Here's how the part is built. I have some questions about the finished solid (model axes, mm). A direction names the side the tool comes from. Coordinates: 2 decimals unless noted, no trailing zeros. Write each loop counter-clockwise with the first axis right and the second up, starting at its lowest first coordinate (ties: lowest second). Pieces come first, ordered by that corner, then holes. Notation, with made-up numbers: M -23,-34 L 8,-34 A27 ccw 8,-4 Z; hole C 11.25,27.25 d5. An arc over 180 degrees is marked long. Use one line per item in the form item = value. Start each with the question number.
1. I want a section at A-A, the plane z = -0.5. List the corners of the cut face in (x, y) for me, plus the area to 3 significant figures.
2. Thinking about a two-plate mould opening in Z: for faces 1 (the face through (-6, 3, -9.5)), 2 (the face through (-6, -3, 1.1)), 3 (the face through (-7.134, -3.724, -8.493)), 4 (the face through (5.95, 4.087, 0.846)), which applies, released by +Z, released by -Z, zero draft, split by the parting line, or undercut?
3. I want a section at B-B, the plane y = 0. List the corners of the cut face in (x, z) for me.
4. On a 3-axis mill with a long thin cutter (end or side, diameter ignored), from which of +Z, -Z, +X, -X, +Y, -Y can I reach the whole of each face in a straight line? I mean faces 5 (the face through (0, -8.2, -6)), 6 (the face through (-5.95, -4.087, 0.846)), 7 (the face through (7.134, -3.724, -0.211)). Say none if no direction works.
5. I want a section at C-C, the plane x = 0. List the corners of the cut face in (y, z) for me, plus the area to 3 significant figures.
6. I'm going to push flat-ended pins straight in: pin 1 Ø1 at (x, z) = (6, -5.5) entering from +Y; pin 2 Ø1.5 at (x, z) = (-3, -5.5) entering from -Y; pin 3 Ø1 at (y, z) = (3, -4) entering from +X. Where does each tip first touch, or does it pass through?
7. I want a section at D-D, the plane z = -4.5. List the corners of the cut face in (x, y) for me.
8. Please list where these lines run through material, in increasing order: line 1 along X through (y, z) = (-0.75, -7.75); line 2 along X through (y, z) = (-2.75, -2.5); line 3 along Y through (x, z) = (4.75, -4). Write a range as [from, to].
from build123d import *

# Parameters (mm, degrees)
SKETCH007_R                    = 8.5
PAD006_DEPTH                   = 7
THICKNESS_T                    = -0.5
PAD007_DEPTH                   = 1.6
PAD007_POLARPATTERN_2_DEPTH    = 1.6
PAD008_DEPTH                   = 0.5
PAD008_POLARPATTERN001_2_DEPTH = 0.5
SKETCH011_W                    = 13.925584
SKETCH011_H                    = 6.6246
POCKET001_DEPTH                = 2
SKETCH013_W                    = 13.925584
SKETCH013_H                    = 6.6246
POCKET002_DEPTH                = 2
SKETCH014_R                    = 8
POCKET003_DEPTH                = 0.5
PAD009_DEPTH                   = 1
PAD009_MIRRORED002_2_DEPTH     = 1
PAD010_DEPTH                   = 0.5
PAD010_MIRRORED004_2_DEPTH     = 0.5
FILLET_R                       = 0.5


with BuildPart() as part:
    # Sketch007 (on DatumPlane) → Pad006 (new body)
    with BuildSketch(Plane(origin=(0, 0, -1), x_dir=(1, 0, 0), z_dir=(0, 0, -1))):
        Circle(SKETCH007_R)
    extrude(amount=PAD006_DEPTH)

    # Thickness
    thickness_openings = [part.faces().sort_by_distance(p)[0] for p in [
        (0, 0, -1),
    ]]
    offset(amount=THICKNESS_T, openings=thickness_openings)

    # Sketch008 (on Face3 of Thickness) → Pad007 (join)
    with BuildSketch(Plane.XY.offset(-1)):
        with BuildLine():
            ThreePointArc((-7.005526, 4.813794), (-7.541696, 3.920819), (-7.964623, 2.96897))
            Line((-7.540357, 2.810816), (-7.964623, 2.96897))
            ThreePointArc((-6.632349, 4.557368), (-7.139959, 3.711961), (-7.540357, 2.810816))
            Line((-6.632349, 4.557368), (-7.005526, 4.813794))
        make_face()
    pad007 = extrude(amount=PAD007_DEPTH)

    # Sketch008 PolarPattern 2 → Pad007 PolarPattern 2 (add)
    with BuildSketch(Plane(origin=(0, 0, -1), x_dir=(-1, 0, 0), z_dir=(0, 0, 1))):
        with BuildLine():
            ThreePointArc((-7.005526, 4.813794), (-7.541696, 3.920819), (-7.964623, 2.96897))
            Line((-7.540357, 2.810816), (-7.964623, 2.96897))
            ThreePointArc((-6.632349, 4.557368), (-7.139959, 3.711961), (-7.540357, 2.810816))
            Line((-6.632349, 4.557368), (-7.005526, 4.813794))
        make_face()
    pad007_polarpattern_2 = extrude(amount=PAD007_POLARPATTERN_2_DEPTH)

    # Mirrored: Pad007, Pad007 PolarPattern 2 across Sketch008 V_Axis
    add(pad007.mirror(Plane(origin=(0, 0, -1), x_dir=(0, 0, 1), z_dir=(1, 0, 0))))
    add(pad007_polarpattern_2.mirror(Plane(origin=(0, 0, -1), x_dir=(0, 0, 1), z_dir=(1, 0, 0))))

    # Sketch009 (on Face23 of MultiTransform) → Pad008 (join)
    with BuildSketch(Plane.XY.offset(0.6)):
        with BuildLine():
            ThreePointArc((-7.005526, 4.813794), (-7.542066, 3.921011), (-7.964623, 2.96897))
            Line((-5.09111, 1.862853), (-7.964623, 2.96897))
            ThreePointArc((-4.469489, 3.068188), (-4.818529, 2.485236), (-5.09111, 1.862853))
            Line((-7.005526, 4.813794), (-4.469489, 3.068188))
        make_face()
    pad008 = extrude(amount=PAD008_DEPTH)

    # Sketch009 PolarPattern001 2 → Pad008 PolarPattern001 2 (add)
    with BuildSketch(Plane(origin=(0, 0, 0.6), x_dir=(-1, 0, 0), z_dir=(0, 0, 1))):
        with BuildLine():
            ThreePointArc((-7.005526, 4.813794), (-7.542066, 3.921011), (-7.964623, 2.96897))
            Line((-5.09111, 1.862853), (-7.964623, 2.96897))
            ThreePointArc((-4.469489, 3.068188), (-4.818529, 2.485236), (-5.09111, 1.862853))
            Line((-7.005526, 4.813794), (-4.469489, 3.068188))
        make_face()
    pad008_polarpattern001_2 = extrude(amount=PAD008_POLARPATTERN001_2_DEPTH)

    # Mirrored001: Pad008, Pad008 PolarPattern001 2 across Sketch009 V_Axis
    add(pad008.mirror(Plane(origin=(0, 0, 0.6), x_dir=(0, 0, 1), z_dir=(1, 0, 0))))
    add(pad008_polarpattern001_2.mirror(Plane(origin=(0, 0, 0.6), x_dir=(0, 0, 1), z_dir=(1, 0, 0))))

    # Sketch011 (on Face1 of ShapeBinder001) → Pocket001 (cut)
    with BuildSketch(Plane(origin=(0, 0, -1), x_dir=(1, 0, 0), z_dir=(0, 0, -1))):
        with Locations((0, 8.1877)):
            Rectangle(SKETCH011_W, SKETCH011_H)
    extrude(amount=POCKET001_DEPTH, mode=Mode.SUBTRACT)

    # Sketch013 → Pocket002 (cut)
    with BuildSketch(Plane.XY.offset(-8)):
        with Locations((0, -8.1877)):
            Rectangle(SKETCH013_W, SKETCH013_H)
    extrude(amount=POCKET002_DEPTH, mode=Mode.SUBTRACT)

    # Sketch014 → Pocket003 (cut)
    with BuildSketch(Plane.XY.offset(-8)):
        Circle(SKETCH014_R)
    extrude(amount=POCKET003_DEPTH, mode=Mode.SUBTRACT)

    # Sketch012 → Pad009 (join)
    with BuildSketch(Plane.XY.offset(-8)):
        with BuildLine():
            ThreePointArc((-7.005526, 4.813794), (-7.541696, 3.920819), (-7.964623, 2.96897))
            Line((-7.540357, 2.810816), (-7.964623, 2.96897))
            ThreePointArc((-6.632349, 4.557368), (-7.139959, 3.711961), (-7.540357, 2.810816))
            Line((-6.632349, 4.557368), (-7.005526, 4.813794))
        make_face()
    pad009 = extrude(amount=-PAD009_DEPTH)

    # Sketch012 Mirrored002 2 → Pad009 Mirrored002 2 (add)
    with BuildSketch(Plane(origin=(0, 0, -8), x_dir=(-1, 0, 0), z_dir=(0, 0, -1))):
        with BuildLine():
            ThreePointArc((-7.005526, 4.813794), (-7.541696, 3.920819), (-7.964623, 2.96897))
            Line((-7.540357, 2.810816), (-7.964623, 2.96897))
            ThreePointArc((-6.632349, 4.557368), (-7.139959, 3.711961), (-7.540357, 2.810816))
            Line((-6.632349, 4.557368), (-7.005526, 4.813794))
        make_face()
    pad009_mirrored002_2 = extrude(amount=PAD009_MIRRORED002_2_DEPTH)

    # Mirrored003: Pad009, Pad009 Mirrored002 2 across Sketch012 H_Axis
    add(pad009.mirror(Plane(origin=(0, 0, -8), x_dir=(0, 0, 1), z_dir=(0, 1, 0))))
    add(pad009_mirrored002_2.mirror(Plane(origin=(0, 0, -8), x_dir=(0, 0, 1), z_dir=(0, 1, 0))))

    # Sketch015 → Pad010 (join)
    with BuildSketch(Plane.XY.offset(-9.5)):
        with BuildLine():
            ThreePointArc((-7.005526, 4.813794), (-7.542066, 3.921011), (-7.964623, 2.96897))
            Line((-5.09111, 1.862853), (-7.964623, 2.96897))
            ThreePointArc((-4.469489, 3.068188), (-4.818529, 2.485236), (-5.09111, 1.862853))
            Line((-7.005526, 4.813794), (-4.469489, 3.068188))
        make_face()
    pad010 = extrude(amount=PAD010_DEPTH)

    # Sketch015 Mirrored004 2 → Pad010 Mirrored004 2 (add)
    with BuildSketch(Plane(origin=(0, 0, -9.5), x_dir=(-1, 0, 0), z_dir=(0, 0, -1))):
        with BuildLine():
            ThreePointArc((-7.005526, 4.813794), (-7.542066, 3.921011), (-7.964623, 2.96897))
            Line((-5.09111, 1.862853), (-7.964623, 2.96897))
            ThreePointArc((-4.469489, 3.068188), (-4.818529, 2.485236), (-5.09111, 1.862853))
            Line((-7.005526, 4.813794), (-4.469489, 3.068188))
        make_face()
    pad010_mirrored004_2 = extrude(amount=-PAD010_MIRRORED004_2_DEPTH)

    # Mirrored005: Pad010, Pad010 Mirrored004 2 across Sketch015 H_Axis
    add(pad010.mirror(Plane(origin=(0, 0, -9.5), x_dir=(0, 0, 1), z_dir=(0, 1, 0))))
    add(pad010_mirrored004_2.mirror(Plane(origin=(0, 0, -9.5), x_dir=(0, 0, 1), z_dir=(0, 1, 0))))

    # Fillet
    fillet_edges = [part.edges().sort_by_distance(p)[0] for p in [
        (-4.469489, 3.068188, 0.85),
        (-5.09111, 1.862853, 0.85),
        (-5.09111, -1.862853, 0.85),
        (-4.469489, -3.068188, 0.85),
        (4.469489, 3.068188, 0.85),
        (5.09111, 1.862853, 0.85),
        (5.09111, -1.862853, 0.85),
        (4.469489, -3.068188, 0.85),
        (-4.469489, 3.068188, -9.25),
        (-5.09111, 1.862853, -9.25),
        (4.469489, 3.068188, -9.25),
        (5.09111, 1.862853, -9.25),
        (-5.09111, -1.862853, -9.25),
        (-4.469489, -3.068188, -9.25),
        (5.09111, -1.862853, -9.25),
        (4.469489, -3.068188, -9.25),
    ]]
    fillet(fillet_edges, radius=FILLET_R)


solid = part.part
Answer list:
q1.outline = M -7.96,-2.97 A8.5 ccw -7.01,-4.81 L -6.63,-4.56 A8.05 cw -7.54,-2.81 Z; M -7.96,2.97 L -7.54,2.81 A8.05 cw -6.63,4.56 L -7.01,4.81 A8.5 ccw Z; M 6.63,-4.56 L 7.01,-4.81 A8.5 ccw 7.96,-2.97 L 7.54,-2.81 A8.05 cw Z; M 6.63,4.56 A8.05 cw 7.54,2.81 L 7.96,2.97 A8.5 ccw 7.01,4.81 Z
q1.area = 3.67 mm²
q2.face_1 = released by -Z
q2.face_2 = released by +Z
q2.face_3 = undercut
q2.face_4 = zero draft
q3.outline = M -8.5,-8 L -8,-8 L -8,-1 L -8.5,-1 Z; M 8,-8 L 8.5,-8 L 8.5,-1 L 8,-1 Z
q4.face_5 = -Z, +X, -X, -Y
q4.face_6 = +Z, -Y
q4.face_7 = none
q5.outline = M -8.5,-6 L -8,-6 L -8,-3 L -8.5,-3 Z; M 8,-8 L 8.5,-8 L 8.5,-1 L 8,-1 Z
q5.area = 5.00 mm²
q6.pin_1 = 6.48
q6.pin_2 = -8.2
q6.pin_3 = 8.12
q7.outline = C 0,0 d17; hole C 0,0 d16
q8.line_1 = [-8.47, -7.96], [7.96, 8.47]
q8.line_2 = [-8.04, -7.51], [7.51, 8.04]
q8.line_3 = [-7.05, -6.44], [6.44, 7.05]
